Design review of the part built by this model. Coordinates are the model's own, in mm. Coordinates: 2 decimals unless noted, no trailing zeros. Loops run counter-clockwise (first coordinate to the right, second up) from the corner with the lowest first, then second, coordinate; pieces in that order, holes last. Notation, with made-up numbers: (86.25, -30.75) -> (122.25, -30.75) arc R32 cw to (122.25, -0.75) -> close; hole circle Ø3 at (-18, 65.5). An arc over 180 degrees is marked (long way). Answer as a JSON object with one key per item and string values.
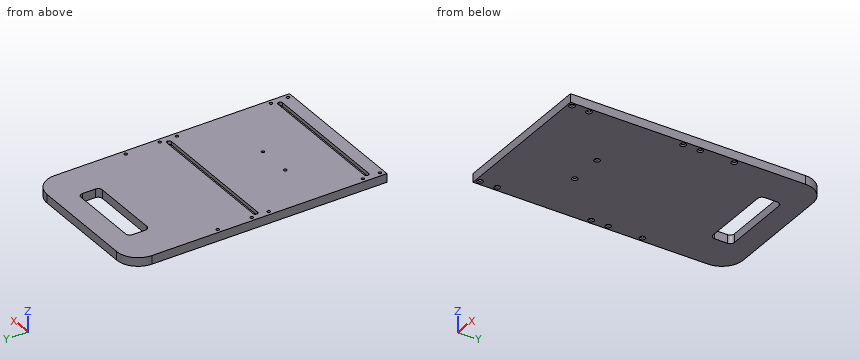
```python
from build123d import *

# Parameters (mm, degrees)
SKETCH1_W                                         = 222.25
SKETCH1_H                                         = 381
BOSS_EXTRUDE1_DEPTH                               = 12.7
FILLET1_R                                         = 31.75
SKETCH2_W                                         = 114.3
SKETCH2_H                                         = 31.75
CUT_EXTRUDE1_DEPTH                                = 12.7
FILLET2_R                                         = 6.35
SKETCH3_W                                         = 203.2
SKETCH3_H                                         = 6.604
CUT_EXTRUDE2_DEPTH                                = 5.334
FILLET3_R                                         = 3.302
CSK_FOR_8_FLAT_HEAD_MACHINE_SCREW_100_D           = 4.4958
CSK_FOR_8_FLAT_HEAD_MACHINE_SCREW_100_CSINK_D     = 8.4328
CSK_FOR_8_FLAT_HEAD_MACHINE_SCREW_100_CSINK_ANGLE = 100


with BuildPart() as part:
    # Sketch1 → Boss-Extrude1 (new body)
    with BuildSketch(Plane.XY):
        Rectangle(SKETCH1_W, SKETCH1_H)
    extrude(amount=BOSS_EXTRUDE1_DEPTH)

    # Fillet1
    fillet1_edges = [part.edges().sort_by_distance(p)[0] for p in [
        (111.125, 190.5, 6.35),
        (-111.125, 190.5, 6.35),
    ]]
    fillet(fillet1_edges, radius=FILLET1_R)

    # Sketch2 → Cut-Extrude1 (cut)
    with BuildSketch(Plane.XY.offset(12.7)):
        with Locations((0, 142.875)):
            Rectangle(SKETCH2_W, SKETCH2_H)
    extrude(amount=-CUT_EXTRUDE1_DEPTH, mode=Mode.SUBTRACT)

    # Fillet2
    fillet2_edges = [part.edges().sort_by_distance(p)[0] for p in [
        (57.15, 127, 6.35),
        (57.15, 158.75, 6.35),
        (-57.15, 158.75, 6.35),
        (-57.15, 127, 6.35),
    ]]
    fillet(fillet2_edges, radius=FILLET2_R)

    # Sketch3 → Cut-Extrude2 (cut)
    with BuildSketch(Plane.XY.offset(12.7)):
        with Locations((0, -168.402)):
            Rectangle(SKETCH3_W, SKETCH3_H)
        with Locations((0, -3.302)):
            Rectangle(SKETCH3_W, SKETCH3_H)
    extrude(amount=-CUT_EXTRUDE2_DEPTH, mode=Mode.SUBTRACT)

    # Fillet3
    fillet3_edges = [part.edges().sort_by_distance(p)[0] for p in [
        (101.6, -165.1, 10.033),
        (101.6, -171.704, 10.033),
        (-101.6, -171.704, 10.033),
        (-101.6, -165.1, 10.033),
        (101.6, -6.604, 10.033),
        (101.6, 0, 10.033),
        (-101.6, 0, 10.033),
        (-101.6, -6.604, 10.033),
    ]]
    fillet(fillet3_edges, radius=FILLET3_R - 0.0001)  # a hair under: the kernel refuses the full size

    # CSK for #8 Flat Head Machine Screw (100)1 (through all)
    with Locations(Plane(origin=(0, 0, 0), x_dir=(-1, 0, 0), z_dir=(0, 0, -1))):
        with Locations((-104.775, -184.15), (-104.775, -158.75), (104.775, -158.75), (104.775, -184.15), (-104.775, -19.05), (-104.775, 6.35), (104.775, 6.35), (104.775, -19.05), (-104.775, 57.15), (104.775, 57.15), (-15.875, -88.9), (34.925, -88.9)):
            CounterSinkHole(CSK_FOR_8_FLAT_HEAD_MACHINE_SCREW_100_D / 2, CSK_FOR_8_FLAT_HEAD_MACHINE_SCREW_100_CSINK_D / 2, counter_sink_angle=CSK_FOR_8_FLAT_HEAD_MACHINE_SCREW_100_CSINK_ANGLE)


solid = part.part
```
1) Add section B-B, the plane z = 4. Count the separate pieces of the cut face and the enclosed holes in it, and give its area (3 significant figures).
Completed:
{"separate pieces": "1", "enclosed holes": "13", "area": "80,500 mm²"}
2) Clearance check with flat-ended pins moving along their axes: pin 1 Ø5.5 at (x, y) = (-43, -170) entering from +Z; pin 2 Ø2 at (x, y) = (10, -2) entering from +Z. State where each tip first meets the part, or that it passes through.
Completed:
{"pin 1": "z = 12.7", "pin 2": "z = 7.37"}
3) Wall thickness on probe 1 along Y at (x, z) = (-47, 7.75); probe 2 along Y at (x, z) = (-77.5, 10.75); probe 3 along X at (y, z) = (-88.9, 4) (3 decimals): over which ranges is each line inside the solid? List them lowest first.
Completed:
{"probe 1": "-190.5 to -171.7, -165.1 to -6.6, 0 to 127, 158.75 to 190.5", "probe 2": "-190.5 to -171.7, -165.1 to -6.6, 0 to 190.5", "probe 3": "-111.125 to -37.173, -32.677 to 13.627, 18.123 to 111.125"}
4) Add section A-A, the plane x = -12. Give the boundary of the cut face in (y, z).
Completed:
{"outline": "(-190.5, 0) -> (127, 0) -> (127, 12.7) -> (0, 12.7) -> (0, 7.37) -> (-6.6, 7.37) -> (-6.6, 12.7) -> (-165.1, 12.7) -> (-165.1, 7.37) -> (-171.7, 7.37) -> (-171.7, 12.7) -> (-190.5, 12.7) -> close; (158.75, 0) -> (190.5, 0) -> (190.5, 12.7) -> (158.75, 12.7) -> close"}
5) Add section C-C, the plane x = -83. Give the boundary of the cut face in (y, z), and give its area (3 significant figures).
Completed:
{"outline": "(-190.5, 0) -> (190.29, 0) -> (190.29, 12.7) -> (0, 12.7) -> (0, 7.37) -> (-6.6, 7.37) -> (-6.6, 12.7) -> (-165.1, 12.7) -> (-165.1, 7.37) -> (-171.7, 7.37) -> (-171.7, 12.7) -> (-190.5, 12.7) -> close", "area": "4,770 mm²"}
